from build123d import *

# Parameters (mm, degrees)
SKETCH_2_W      = 6
SKETCH_2_H      = 6
EXTRUDE_1_DEPTH = 20


with BuildPart() as part:
    # 草图1 → 旋转1 (revolve)
    with BuildSketch(Plane.XY, mode=Mode.PRIVATE) as revolve_1_sk:
        with BuildLine():
            Line((-5, 9.572809864), (-5, 11.128838899))
            Line((-5, 11.128838899), (-3.694047059, 11.128838899))
            Line((-3.694047059, 11.128838899), (0, 11.128838899))
            Line((0, 11.128838899), (0, -6))
            ThreePointArc((0, -6), (-5.889524943, -1.146078506), (-2.249952649, 5.56216802))
            ThreePointArc((-2.249952649, 5.56216802), (-1.71510176, 6.07424335), (-1.67910561, 6.813831678))
            add(Edge.make_bspline(
                [(-1.67910561, 6.813831678), (-2.255406993, 8.492909128), (-5, 9.572809864)],
                knots=[0, 0, 0, 1, 1, 1], degree=2))
        make_face()
    revolve(revolve_1_sk.sketch.rotate(Axis((0, 11.882352941, 0), (0, -1, 0)), 270), axis=Axis((0, 11.882352941, 0), (0, -1, 0)))

    # 草图2 → 凸台-拉伸1 (add)
    with BuildSketch(Plane(origin=(0, 11.128838899, 0), x_dir=(1, 0, 0), z_dir=(0, 1, 0))):
        Rectangle(SKETCH_2_W, SKETCH_2_H)
    extrude(amount=EXTRUDE_1_DEPTH)


solid = part.part
Design review of the part built by this model. Coordinates are the model's own, in mm. A direction names the side the tool comes from. Give positions to 0.01 mm unless a question says otherwise; leave off trailing zeros. Write each loop counter-clockwise with the first axis right and the second up, starting at its lowest first coordinate (ties: lowest second). Pieces come first, ordered by that corner, then holes. Notation, with made-up numbers: M -2.75,-9.75 L 47.25,-9.75 A15 cw 47.25,14.25 Z; hole C 82.5,59.5 d9. An arc over 180 degrees is marked long. Return JSON: item names as keys, results as strings. Group by question number.
Item 1: Take a section at A-A (y = 22). Give the boundary of the cut face in (x, z).
Item 2: Take a section at C-C (y = 3). Give the boundary of the cut face in (x, z), plus the area to 3 significant figures.
Item 3: Clearance check with flat-ended pins moving along their axes: pin 1 Ø3 at (y, z) = (20, 3.5) entering from +X; pin 2 Ø5 at (y, z) = (20.5, -1) entering from -X; pin 3 Ø4 at (x, z) = (-2.5, 2.5) entering from -Y. State where each tip first meets the part, or that it passes through.
Item 4: Tool access review of faces 1 (the cylindrical face through (4.88, 10.36, -1.08)), 2 (the flat face through (0, 21, 3)), 3 (the flat face through (-3, 21, 0)): name each direction out of +Z, -Z, +X, -X, +Y, -Y from which nothing blocks a thin tool from reaching the whole face with its end or side.
Item 5: Wall thickness on line 1 along Y through (x, z) = (1.5, 3.5); line 2 along X through (y, z) = (22.5, 1.75); line 3 along Y through (x, z) = (-2.25, 0.25): over which ranges is each line inside the solid? List them lowest first.
Item 6: Take a section at B-B (y = 10). Give the boundary of the cut face in (x, z), plus the area to 3 significant figures.
Return value:
{
 "1": {"outline": "M -3,-3 L 3,-3 L 3,3 L -3,3 Z"},
 "2": {"outline": "C 0,0 d10.39", "area": "84.8 mm2"},
 "3": {"pin 1": "stops at x = 3", "pin 2": "stops at x = -3", "pin 3": "stops at y = -5.8"},
 "4": {"face 1": "+Y", "face 2": "+Z, +X, -X, +Y", "face 3": "+Z, -Z, -X, +Y"},
 "5": {"line 1": "y = -4.64 to 4.64, 9.02 to 11.13", "line 2": "x = -3 to 3", "line 3": "y = -5.56 to 5.56, 7.82 to 31.13"},
 "6": {"outline": "C 0,0 d10", "area": "78.5 mm2"}
}
